Here's how the part is built. I have some questions about the finished solid (model axes, mm). A direction names the side the tool comes from. Round coordinates to 2 decimals unless told otherwise and drop trailing zeros. Write each loop counter-clockwise with the first axis right and the second up, starting at its lowest first coordinate (ties: lowest second). Pieces come first, ordered by that corner, then holes. Notation, with made-up numbers: (-8, 9.25) -> (-1, 9.25) arc R15 cw to (-1, 17.25) -> close; hole circle Ø10 at (67.25, -9). An arc over 180 degrees is marked (long way). Answer as CSV lines item,"result".
from build123d import *

# Parameters (mm, degrees)
FILLET1_R                       = 0.5
BOSS_EXTRUDE6_REACH             = 33.084
BOSS_EXTRUDE6_DIRECTION_2_REACH = 33.084
MIRROR2_COPY_1_REACH            = 33.084
MIRROR2_COPY_2_REACH            = 33.084


with BuildPart() as part:
    # Sweep1: sweep along a path in Sketch2path
    with BuildLine(Plane.XY) as sweep1_path:
        Line((0, 0), (25, 0))
    # Sketch3 → Sweep1 (sweep)
    with BuildSketch(Plane(origin=(0, 0, 0), x_dir=(0, 0, -1), z_dir=(1, 0, 0))):
        with BuildLine():
            Line((12.65, 8), (-12.65, 8))
            ThreePointArc((-12.65, 8), (-15.478427125, 6.828427125), (-16.65, 4))
            Line((-16.65, 4), (-16.65, -4))
            ThreePointArc((-16.65, -4), (-15.478427125, -6.828427125), (-12.65, -8))
            Line((-12.65, -8), (12.65, -8))
            ThreePointArc((12.65, -8), (15.478427125, -6.828427125), (16.65, -4))
            Line((16.65, -4), (16.65, 4))
            ThreePointArc((16.65, 4), (15.478427125, 6.828427125), (12.65, 8))
        make_face()
        with BuildLine():
            Line((-15.65, 4), (-15.65, -4))
            ThreePointArc((-15.65, -4), (-14.771320344, -6.121320344), (-12.65, -7))
            Line((-12.65, -7), (12.65, -7))
            ThreePointArc((12.65, -7), (14.771320344, -6.121320344), (15.65, -4))
            Line((15.65, -4), (15.65, 4))
            ThreePointArc((15.65, 4), (14.771320344, 6.121320344), (12.65, 7))
            Line((12.65, 7), (-12.65, 7))
            ThreePointArc((-12.65, 7), (-14.771320344, 6.121320344), (-15.65, 4))
        make_face(mode=Mode.SUBTRACT)
    sweep(path=sweep1_path.line)

    # Fillet1
    fillet1_edges = [part.edges().sort_by_distance(p)[0] for p in [
        (25, 6.121320344, -14.771320344),
        (25, 0, -15.65),
        (25, -6.121320344, -14.771320344),
        (0, 0, 15.65),
        (0, -6.121320344, 14.771320344),
        (0, -7, 0),
        (0, -6.121320344, -14.771320344),
        (0, 0, -15.65),
        (0, 6.121320344, -14.771320344),
        (25, -7, 0),
        (0, 7, 0),
        (0, 6.121320344, 14.771320344),
        (25, -6.121320344, 14.771320344),
        (25, 0, 15.65),
        (25, 6.121320344, 14.771320344),
        (25, 7, 0),
    ]]
    fillet(fillet1_edges, radius=FILLET1_R)

    # Sketch13 → Boss-Extrude6 (add, up to next)
    with BuildSketch(Plane(origin=(0, 0, 0), x_dir=(1, 0, 0), z_dir=(0, 1, 0)), mode=Mode.PRIVATE) as boss_extrude6_sk1:
        with BuildLine():
            Line((15.99, -6), (16.01, -6))
            ThreePointArc((16.01, -6), (17.417142495, -6.582857505), (18, -7.99))
            Line((18, -7.99), (18, -10))
            Line((18, -10), (14, -10))
            Line((14, -10), (14, -7.99))
            ThreePointArc((14, -7.99), (14.582857505, -6.582857505), (15.99, -6))
        make_face()
    boss_extrude6_tool1 = extrude(boss_extrude6_sk1.sketch, amount=BOSS_EXTRUDE6_REACH, mode=Mode.PRIVATE) - part.part
    boss_extrude6 = boss_extrude6_tool1.solids().sort_by_distance((16, 0, 8.184882))[0]
    add(boss_extrude6)

    # Sketch13 → Boss-Extrude6 direction 2 (add, up to next)
    with BuildSketch(Plane(origin=(0, 0, 0), x_dir=(1, 0, 0), z_dir=(0, 1, 0)), mode=Mode.PRIVATE) as boss_extrude6_direction_2_sk1:
        with BuildLine():
            Line((15.99, -6), (16.01, -6))
            ThreePointArc((16.01, -6), (17.417142495, -6.582857505), (18, -7.99))
            Line((18, -7.99), (18, -10))
            Line((18, -10), (14, -10))
            Line((14, -10), (14, -7.99))
            ThreePointArc((14, -7.99), (14.582857505, -6.582857505), (15.99, -6))
        make_face()
    boss_extrude6_direction_2_tool1 = extrude(boss_extrude6_direction_2_sk1.sketch, amount=-BOSS_EXTRUDE6_DIRECTION_2_REACH, mode=Mode.PRIVATE) - part.part
    boss_extrude6_direction_2 = boss_extrude6_direction_2_tool1.solids().sort_by_distance((16, 0, 8.184882))[0]
    add(boss_extrude6_direction_2)

    # Mirror1: Boss-Extrude6, Boss-Extrude6 direction 2 across plane
    add(boss_extrude6.mirror(Plane(origin=(12.5, 0, 0), x_dir=(0, 0, 1), z_dir=(1, 0, 0))))
    add(boss_extrude6_direction_2.mirror(Plane(origin=(12.5, 0, 0), x_dir=(0, 0, 1), z_dir=(1, 0, 0))))

    # Mirror2: Boss-Extrude6, Boss-Extrude6 direction 2 across plane
    add(boss_extrude6.mirror(Plane.XY))
    add(boss_extrude6_direction_2.mirror(Plane.XY))

    # Mirror2 copy 1 sketch → Mirror2 copy 1 (add, up to next)
    with BuildSketch(Plane(origin=(25, 0, 0), x_dir=(-1, 0, 0), z_dir=(0, 1, 0)), mode=Mode.PRIVATE) as mirror2_copy_1_sk1:
        with BuildLine():
            Line((15.99, -6), (16.01, -6))
            ThreePointArc((16.01, -6), (17.417142495, -6.582857505), (18, -7.99))
            Line((18, -7.99), (18, -10))
            Line((18, -10), (14, -10))
            Line((14, -10), (14, -7.99))
            ThreePointArc((14, -7.99), (14.582857505, -6.582857505), (15.99, -6))
        make_face()
    mirror2_copy_1_tool1 = extrude(mirror2_copy_1_sk1.sketch, amount=MIRROR2_COPY_1_REACH, mode=Mode.PRIVATE) - part.part
    add(mirror2_copy_1_tool1.solids().sort_by_distance((9, 0, -8.184882))[0])

    # Mirror2 copy 2 sketch → Mirror2 copy 2 (add, up to next)
    with BuildSketch(Plane(origin=(25, 0, 0), x_dir=(-1, 0, 0), z_dir=(0, 1, 0)), mode=Mode.PRIVATE) as mirror2_copy_2_sk1:
        with BuildLine():
            Line((15.99, -6), (16.01, -6))
            ThreePointArc((16.01, -6), (17.417142495, -6.582857505), (18, -7.99))
            Line((18, -7.99), (18, -10))
            Line((18, -10), (14, -10))
            Line((14, -10), (14, -7.99))
            ThreePointArc((14, -7.99), (14.582857505, -6.582857505), (15.99, -6))
        make_face()
    mirror2_copy_2_tool1 = extrude(mirror2_copy_2_sk1.sketch, amount=-MIRROR2_COPY_2_REACH, mode=Mode.PRIVATE) - part.part
    add(mirror2_copy_2_tool1.solids().sort_by_distance((9, 0, -8.184882))[0])


solid = part.part
Item 1: Suppose I cut it at A-A, the plane z = -9. List the corners of the cut face in (x, y) for me, then the cut area to 3 significant figures.
Results found:
outline,"(0, -8) -> (25, -8) -> (25, -7.5) arc R0.5 ccw to (24.5, -7) -> (18, -7) -> (18, 7) -> (24.5, 7) arc R0.5 ccw to (25, 7.5) -> (25, 8) -> (0, 8) -> (0, 7.5) arc R0.5 ccw to (0.5, 7) -> (7, 7) -> (7, -7) -> (0.5, -7) arc R0.5 ccw to (0, -7.5) -> close; hole (11, -7) -> (14, -7) -> (14, 7) -> (11, 7) -> close"
area,"162 mm²"
Item 2: If we mould it in two halves opening along X, with no side actions, what happens to faces 6 (the cylindrical face through (7.598, 0.098, -6.567)), 7 (the flat face through (14, 0, -9)), 8 (the flat face through (13, 0, 15.65))? For each: pulls with the +X half, pulls with the -X half, needs draft (parallel to the pull), parting line crosses it, or undercut.
Results found:
face 6,"pulls with the -X half"
face 7,"undercut"
face 8,"needs draft"
Item 3: I need wall thicknesses on L1, parallel to Z at x = 18.25, y = 3.5; L2, parallel to Y at x = 11.25, z = 9; L3, parallel to Z at x = 9, y = 5. Which ranges of each line are inside material? Lowest first, please.
Results found:
L1,"z = -16.65 to -15.65, 15.65 to 16.65"
L2,"y = -8 to -7, 7 to 8"
L3,"z = -16.52 to -15.48, -10 to -6, 6 to 10, 15.48 to 16.52"
Item 4: Suppose I cut it at D-D, the plane y = -3.5. State how many separate pieces and enclosed holes the cut face has, then the cut area to 3 significant figures.
Results found:
separate pieces,"6"
enclosed holes,"0"
area,"107 mm²"
Item 5: Suppose I cut it at B-B, the plane x = 6. List the corners of the cut face in (y, z) for me, then the cut area to 3 significant figures.
Results found:
outline,"(-8, -12.65) arc R4 ccw to (-4, -16.65) -> (4, -16.65) arc R4 ccw to (8, -12.65) -> (8, 12.65) arc R4 ccw to (4, 16.65) -> (-4, 16.65) arc R4 ccw to (-8, 12.65) -> close; hole (-7, -12.65) arc R3 ccw to (-4, -15.65) -> (4, -15.65) arc R3 ccw to (7, -12.65) -> (7, 12.65) arc R3 ccw to (4, 15.65) -> (-4, 15.65) arc R3 ccw to (-7, 12.65) -> close"
area,"88.6 mm²"
Item 6: For faces 1 (the cylindrical face through (12.67, 6.14, 14.75)), 2 (the cylindrical face through (14.567, 0.098, 6.598)), 3 (the flat face through (18, 0, -9)), 4 (the flat face through (13, 0, 16.65)), 5 (the flat face through (7, 0, 9)), which set-ups out of +Z, -Z, +X, -X, +Y, -Y let a thin tool reach every point of the face, with its end or its side?
Results found:
face 1,"+X, -X"
face 2,"none"
face 3,"+X"
face 4,"+Z, +X, -X, +Y, -Y"
face 5,"-X"
Item 7: Will these pins go through, and if not, where does the flat tip stop? pin 1 (2 mm diameter, centred on y = -3, z = -9, fed in from -X); pin 2 (0.6 mm diameter, centred on y = -2.5, z = 9.5, fed in from +X); pin 3 (1 mm diameter, centred on x = 21, y = -6, fed in from -Z).
Results found:
pin 1,"stops at x = 7"
pin 2,"stops at x = 18"
pin 3,"stops at z = -16.36"
Item 8: Suppose I cut it at C-C, the plane z = 2. List the corners of the cut face in (x, y) for me, then the cut area to 3 significant figures.
Results found:
outline,"(0, -8) -> (25, -8) -> (25, -7.5) arc R0.5 ccw to (24.5, -7) -> (0.5, -7) arc R0.5 ccw to (0, -7.5) -> close; (0, 7.5) arc R0.5 ccw to (0.5, 7) -> (24.5, 7) arc R0.5 ccw to (25, 7.5) -> (25, 8) -> (0, 8) -> close"
area,"49.8 mm²"
